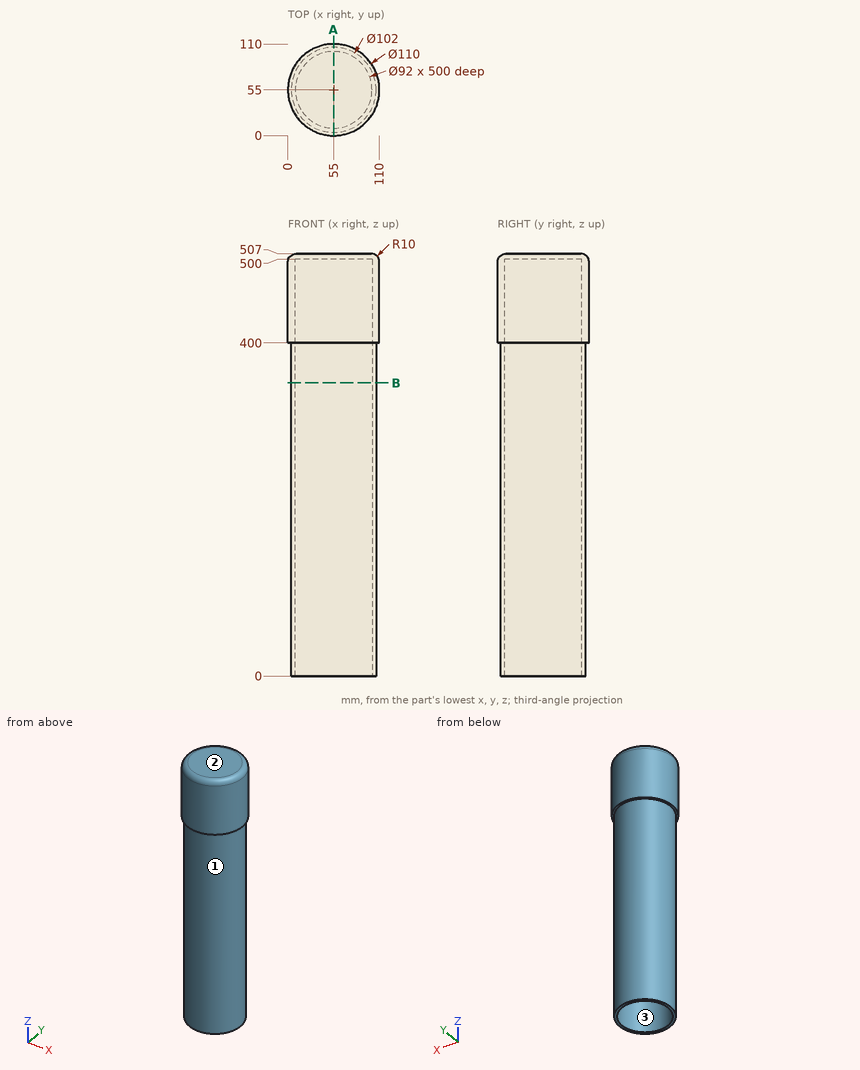
Drawing for the job (mm, zero at the part's lowest x, y, z). Round coordinates to 2 decimals unless told otherwise and drop trailing zeros. Order: outer loops, then holes, each group sorted by start corner. A loop starts at its lowest first (then second) coordinate and runs counter-clockwise, first axis right, second up. Notation, with made-up numbers: (26, -24.75) -> (63, -24.75) arc R24 ccw to (63, -3.75) -> close; hole circle Ø8 at (3, -29). An arc over 180 degrees is marked (long way). Put each result on its own line as item: value.
Q1. Pin check, flat tips, straight feed: pin 1 Ø1.5 at (x, z) = (79, 179) entering from +Y; pin 2 Ø2 at (y, z) = (98, 143.5) entering from +X; pin 3 Ø12 at (y, z) = (37, 135.5) entering from -X. Stop position of each tip, or through.
From the geometry:
pin 1: stops at y = 100.39
pin 2: stops at x = 83.93
pin 3: stops at x = 5.43
Q2. Wall check: line 1 (Y direction, x = 52, z = 274.5); line 2 (Y direction, x = 55, z = 294); line 3 (X direction, y = 53, z = 352.5). Give the ranges that are in metal, low to high. Write a range as [from, to].
From the geometry:
line 1: y = [4.09, 9.1], [100.9, 105.91]
line 2: y = [4, 9], [101, 106]
line 3: x = [4.04, 9.04], [100.96, 105.96]
Q3. Band-saw the part on B-B (z = 352). Give the cut face in (x, y), and give its area (3 significant figures).
From the geometry:
outline: circle Ø102 at (55, 55); hole circle Ø92 at (55, 55)
area: 1,520 mm2
Q4. Pull direction Y, two halves, no side cores. Call the marked faces 1, 2 and 3: pulls with the +Y half, pulls with the -Y half, needs draft (parallel to the pull), parting line crosses it, or undercut.
From the geometry:
face 1: parting line crosses it
face 2: needs draft
face 3: undercut
Q5. Band-saw the part on A-A (x = 55). Give the cut face in (y, z).
From the geometry:
outline: (0, 400) -> (4, 400) -> (4, 0) -> (9, 0) -> (9, 500) -> (101, 500) -> (101, 0) -> (106, 0) -> (106, 400) -> (110, 400) -> (110, 497) arc R10 ccw to (100, 507) -> (10, 507) arc R10 ccw to (0, 497) -> close
